Study the drawing (mm; zero at the part's minimum x, y, z) and answer. A direction names the side the tool comes from. Round coordinates to 2 decimals unless told otherwise and drop trailing zeros. Order: outer loops, then holes, each group sorted by start corner. A loop starts at its lowest first (then second) coordinate and runs counter-clockwise, first axis right, second up. Notation, with made-up numbers: (8, 26) - (37, 26) arc R14 cw to (37, 34) - close; hole circle Ø7 at (-27, 59.25). An arc over 180 degrees is marked (long way). Put each result on its own line as item: value. Start each with the question number.
Q1. Section B-B on x = 17 is taken. Give the vertices of the cut face in (y, z), then the cut area to 3 significant figures.
Q2. Which of the six approach directions +Z, -Z, +X, -X, +Y, -Y give full straight-line access (tool end or side, diameter ignored) to the marked faces 5 and 6?
Q3. Find the intervals of material crossed by line 1 along Y through (x, z) = (17, 3.5); line 2 along X through (y, z) = (21.5, 1.5) (1 decimal); line 3 along Y through (x, z) = (19, 0.5) (1 decimal), in increasing order. Write a range as from..to.
Q4. For a pull along X with two mould halves and no side action, classify the marked faces 1, 2, 3 and 4 as pulls with the +X half, pulls with the -X half, needs draft (parallel to the pull), parting line crosses it, or undercut.
Q5. Section A-A on z = 2.5 is taken. Give the vertices of the cut face in (x, y).
Q6. Section D-D on z = 5.5 is taken. Give the vertices of the cut face in (x, y), then the cut area to 3 significant figures.
Q7. Each of these flat-tipped pins is pushed along its axis until it touches: pin 1 Ø4 at (x, z) = (23, 6) entering from +Y; pin 2 Ø15 at (x, y) = (21, 17) entering from -Z; pin 3 Ø4 at (x, y) = (28, 21.5) entering from -Z; pin 4 Ø1 at (y, z) = (25, 1.5) entering from -X (1 decimal). Where does it stop, or does it pass through?
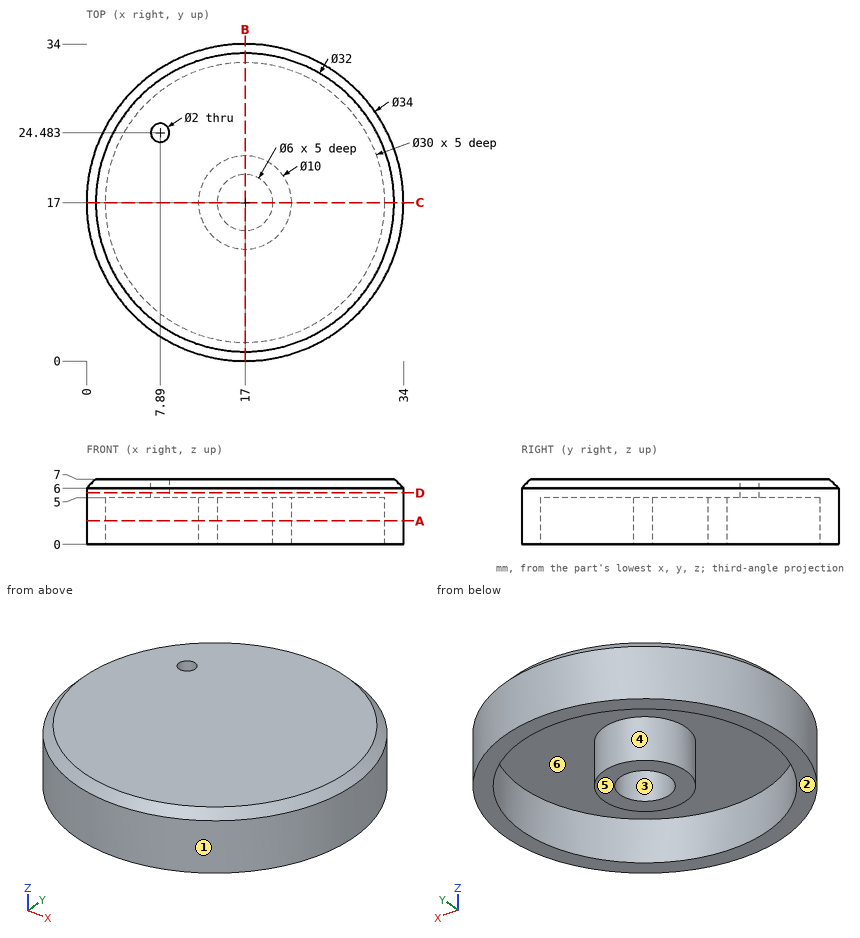
Findings:
1. outline: (0, 0) - (2, 0) - (2, 5) - (12, 5) - (12, 0) - (14, 0) - (14, 5) - (20, 5) - (20, 0) - (22, 0) - (22, 5) - (32, 5) - (32, 0) - (34, 0) - (34, 6) - (33, 7) - (1, 7) - (0, 6) - close
1. area: 107 mm2
2. face 5: -Z, +X, -X, +Y, -Y
2. face 6: -Z
3. line 1: 0..2, 12..14, 20..22, 32..34
3. line 2: 0.6..2.7, 14.8..19.2, 31.3..33.4
3. line 3: 0.1..2.1, 12.4..14.8, 19.2..21.6, 31.9..33.9
4. face 1: parting line crosses it
4. face 2: needs draft
4. face 3: undercut
4. face 4: undercut
5. outline: circle Ø34 at (17, 17); circle Ø10 at (17, 17); hole circle Ø30 at (17, 17); hole circle Ø6 at (17, 17)
6. outline: circle Ø34 at (17, 17); hole circle Ø2 at (7.89, 24.48)
6. area: 905 mm2
7. pin 1: y = 33.52
7. pin 2: z = 0
7. pin 3: z = 5
7. pin 4: x = 1.7
